from build123d import *

# Parameters (mm, degrees)
BOSS_EXTRUDE1_DEPTH = 3.175
SKETCH2_R           = 2.54
CUT_EXTRUDE1_DEPTH  = 4.175
CHAMFER1_SIZE       = 5.08


with BuildPart() as part:
    # Sketch1 → Boss-Extrude1 (new body)
    with BuildSketch(Plane.XY):
        Polygon((-95.364356197, 10.475976437), (-35.039356197, 10.475976437), (-35.039356197, 70.800976437), (-76.314356197, 112.075976437), (-95.364356197, 112.075976437), align=None)
    extrude(amount=BOSS_EXTRUDE1_DEPTH)

    # Sketch2 → Cut-Extrude1 (cut, through all)
    with BuildSketch(Plane(origin=(0, 0, 0), x_dir=(-1, 0, 0), z_dir=(0, 0, -1))):
        with Locations((44.162734276, 20.000976437)):
            Circle(SKETCH2_R)
        with Locations((85.617120669, 20.000976437)):
            Circle(SKETCH2_R)
        with Locations((85.617120669, 61.45536283)):
            Circle(SKETCH2_R)
        with Locations((85.617120669, 102.909749223)):
            Circle(SKETCH2_R)
        with Locations((44.162734276, 61.45536283)):
            Circle(SKETCH2_R)
    extrude(amount=-CUT_EXTRUDE1_DEPTH, mode=Mode.SUBTRACT)

    # Chamfer1
    chamfer1_edges = [part.edges().sort_by_distance(p)[0] for p in [
        (-95.364356197, 112.075976437, 1.5875),
        (-35.039356197, 10.475976437, 1.5875),
        (-95.364356197, 10.475976437, 1.5875),
    ]]
    chamfer(chamfer1_edges, length=CHAMFER1_SIZE)


solid = part.part
Work out the finished part from the listing and answer in its coordinate system (mm). Give positions to 0.01 mm unless a question says otherwise; leave off trailing zeros. Loops run counter-clockwise (first coordinate to the right, second up) from the corner with the lowest first, then second, coordinate; pieces in that order, holes last. Notation, with made-up numbers: (38, -1.5) - (69, -1.5) arc R27 ccw to (69, 30.5) - close; hole circle Ø5 at (36.5, 46). An arc over 180 degrees is marked (long way). Answer in a Markdown table with one row per item. Add a question column.
Q1. The part is cut by section C-C (y = 81.5). Determine the outline of the cut face in (x, z) (3 decimals).
Q2. The part is cut by section B-B (x = -63). Determine the outline of the cut face in (y, z) (3 decimals).
Q3. Determine the mould class of faces 1 (the flat face through (-66, 51, 3.175)), 2 (the flat face through (-95.364, 62, 2)), 3 (the cylindrical face through (-83.6, 18.46, 1.57)), 4 (the cylindrical face through (-46.51, 19.03, 1.57)) for opening direction X: released by +X, released by -X, zero draft, split by the parting line, or undercut.
Q4. This flat-tipped pin is pushed along its axis until it touches: P1, Ø1.5, axis at x = -42.5, z = 2.5, coming from the +Y side. Where does it stop, or does it pass through?
Q5. The part is cut by section A-A (z = 1.95). Determine the outline of the cut face in (x, y).
Q6. Consider line 1 along X through (y, z) = (20, 1.4); line 2 along Y through (x, z) = (-84.5, 1.2); line 3 along Y through (x, z) = (-46.5, 0.8). Determine where each line is inside the solid, lowest interval first.
Solution:
| question | item | result |
|---|---|---|
| 1 | outline | (-95.364, 0) - (-45.738, 0) - (-45.738, 3.175) - (-95.364, 3.175) - close |
| 2 | outline | (10.476, 0) - (98.762, 0) - (98.762, 3.175) - (10.476, 3.175) - close |
| 3 | face 1 | zero draft |
| 3 | face 2 | released by -X |
| 3 | face 3 | undercut |
| 3 | face 4 | undercut |
| 4 | P1 | stops at y = 79.01 |
| 5 | outline | (-95.36, 15.56) - (-90.28, 10.48) - (-40.12, 10.48) - (-35.04, 15.56) - (-35.04, 70.8) - (-76.31, 112.08) - (-90.28, 112.08) - (-95.36, 107) - close; hole circle Ø5.08 at (-85.62, 20); hole circle Ø5.08 at (-85.62, 61.46); hole circle Ø5.08 at (-85.62, 102.91); hole circle Ø5.08 at (-44.16, 20); hole circle Ø5.08 at (-44.16, 61.46) |
| 6 | line 1 | x = -95.36 to -88.16, -83.08 to -46.7, -41.62 to -35.04 |
| 6 | line 2 | y = 10.48 to 17.72, 22.28 to 59.17, 63.74 to 100.63, 105.19 to 112.08 |
| 6 | line 3 | y = 10.48 to 19.01, 21 to 60.46, 62.45 to 82.26 |
